Design review of the part built by this model. Coordinates are the model's own, in mm. A direction names the side the tool comes from. Round coordinates to 2 decimals unless told otherwise and drop trailing zeros. Loops run counter-clockwise (first coordinate to the right, second up) from the corner with the lowest first, then second, coordinate; pieces in that order, holes last. Notation, with made-up numbers: (22.5, 61) - (54.5, 61) arc R6 ccw to (54.5, 68) - close; hole circle Ø6 at (-5, 31.5). An arc over 180 degrees is marked (long way). One line per question, with ' | ' between items. Start each with the question number.
Autodesk Inventor part; units mm, degrees
ref_plane "YZ Plane" through (0, 0, 0) normal (1, 0, 0) x (0, 1, 0)
ref_plane "XZ Plane" through (0, 0, 0) normal (0, 1, 0) x (-1, 0, 0)
ref_plane "XY Plane" through (0, 0, 0) normal (0, 0, 1) x (1, 0, 0)
sketch "Sketch1" plane through (0, 0, 0) normal (0, 0, 1) x (1, 0, 0)
  circle A0 centre (0, 0) radius 18.161
  dimension "d0" = 36.322
extrude "Extrusion1" add sketch "Sketch1" against normal blind 330.2
sketch "Sketch2" plane through (0, 0, 0) normal (0, 0, 1) x (1, 0, 0)
  circle A0 centre (0, 0) radius 18.161
  circle A1 centre (0, 0) radius 12.7
  dimension "d3" = 25.4
extrude "Extrusion2" add sketch "Sketch2" along normal blind 25.4 contours A1
chamfer "Chamfer1" distance 8.89 angle 45 1 edges at (-12.7, 0, 25.4)
properties part number "machineTorchHead"
1. To check wall thickness, follow line 1 along Y through (x, z) = (-1, -70.5); line 2 along Z through (x, y) = (9, -11); line 3 along X through (y, z) = (-13, -237). State the ranges of each line that lie inside material, in increasing order.
2. Clearance check with flat-ended pins moving along their axes: P1, Ø10, axis at y = -9.5, z = -199.5, coming from the -X side; P2, Ø10, axis at x = -4, z = -264, coming from the -Y side; P3, Ø5, axis at x = -1.5, y = 12, coming from the +Z side. State where each tip first meets the part, or that it passes through.
3. Machinability: for faces 1 (the face through (0, 0, 25.4)), 2 (the face through (-2.75, 12.4, 8.14)), which of the approach directions +Z, -Z, +X, -X, +Y, -Y give a long, thin tool a straight path to every point of the face, cutting with its end or side? Answer none if there is none.
4. Take a section at A-A, the plane x = 0. Give the boundary of the cut face in (y, z).
5. Take a section at C-C, the plane z = -268.5. Give the boundary of the cut face in (x, y).
Answer list:
1) line 1: y = -18.13 to 18.13 | line 2: z = -330.2 to 0 | line 3: x = -12.68 to 12.68
2) P1: stops at x = -17.59 | P2: stops at y = -18.16 | P3: stops at z = 19.62
3) face 1: +Z, +X, -X, +Y, -Y | face 2: +Z
4) outline: (-18.16, -330.2) - (18.16, -330.2) - (18.16, 0) - (12.7, 0) - (12.7, 16.51) - (3.81, 25.4) - (-3.81, 25.4) - (-12.7, 16.51) - (-12.7, 0) - (-18.16, 0) - close
5) outline: circle Ø36.32 at (0, 0)
